Geometry check sheet. Reference: the model listing, model coordinates, mm. A direction names the side the tool comes from. Round coordinates to 2 decimals unless told otherwise and drop trailing zeros. Write each loop counter-clockwise with the first axis right and the second up, starting at its lowest first coordinate (ties: lowest second). Pieces come first, ordered by that corner, then holes. Notation, with made-up numbers: (14, 26) -> (22, 26) arc R12 cw to (22, 35) -> close; hole circle Ø8 at (74.5, 26.25). An arc over 180 degrees is marked (long way). Use a Markdown table: item, result.
```python
from build123d import *

# Parameters (mm, degrees)
SKETCH_1_W          = 110
SKETCH_1_H          = 50
EXTRUDE_1_DEPTH     = 6
SKETCH_2_W          = 80
SKETCH_2_H          = 50
EXTRUDE_2_DEPTH     = 34
SKETCH_3_W          = 70
SKETCH_3_H          = 40
CUT_EXTRUDE_1_DEPTH = 28
SKETCH_4_R          = 10
CUT_EXTRUDE_2_DEPTH = 73.456883731
SKETCH_5_R          = 4
CUT_EXTRUDE_3_DEPTH = 111
SKETCH_6_W          = 70
SKETCH_6_H          = 40
CUT_EXTRUDE_4_DEPTH = 6


with BuildPart() as part:
    # 草图1 → 凸台-拉伸1 (new body)
    with BuildSketch(Plane(origin=(0, 0, 0), x_dir=(1, 0, 0), z_dir=(0, 1, 0))):
        Rectangle(SKETCH_1_W, SKETCH_1_H)
    extrude(amount=EXTRUDE_1_DEPTH)

    # 草图2 → 凸台-拉伸2 (add)
    with BuildSketch(Plane(origin=(0, 6, 0), x_dir=(1, 0, 0), z_dir=(0, 1, 0))):
        Rectangle(SKETCH_2_W, SKETCH_2_H)
    extrude(amount=EXTRUDE_2_DEPTH)

    # 草图3 → 切除-拉伸1 (cut)
    with BuildSketch(Plane(origin=(0, 6, 0), x_dir=(1, 0, 0), z_dir=(0, 1, 0))):
        Rectangle(SKETCH_3_W, SKETCH_3_H)
    extrude(amount=CUT_EXTRUDE_1_DEPTH, mode=Mode.SUBTRACT)

    # 草图4 → 切除-拉伸2 (cut, through all)
    with BuildSketch(Plane(origin=(0, 40, 0), x_dir=(1, 0, 0), z_dir=(0, 1, 0))):
        with Locations(Location((0, 0, 0), (0, 0, 270))):
            Circle(SKETCH_4_R)
    extrude(amount=-CUT_EXTRUDE_2_DEPTH, mode=Mode.SUBTRACT)

    # 草图5 → 切除-拉伸3 (cut, symmetric)
    with BuildSketch(Plane(origin=(0, 6, 0), x_dir=(1, 0, 0), z_dir=(0, 1, 0))):
        with Locations(Location((-47.5, 0, 0), (0, 0, 90))):
            Circle(SKETCH_5_R)
        with Locations(Location((47.5, 0, 0), (0, 0, 90))):
            Circle(SKETCH_5_R)
    extrude(amount=CUT_EXTRUDE_3_DEPTH, both=True, mode=Mode.SUBTRACT)

    # 草图6 → 切除-拉伸4 (cut)
    with BuildSketch(Plane(origin=(0, 0, 0), x_dir=(1, 0, 0), z_dir=(0, 1, 0))):
        Rectangle(SKETCH_6_W, SKETCH_6_H)
    extrude(amount=CUT_EXTRUDE_4_DEPTH, mode=Mode.SUBTRACT)


solid = part.part
```
(1) Gauge pin test, flat ends, axial feed: pin 1 Ø20 at (x, z) = (0.5, 5) entering from -Y; pin 2 Ø17 at (y, z) = (18.5, 8.5) entering from +X; pin 3 Ø7.5 at (x, z) = (46, 7) entering from +Y. Record the tip position at first contact, or that the pin passes through.
A:
| item | result |
|---|---|
| pin 1 | stops at y = 34 |
| pin 2 | stops at x = 40 |
| pin 3 | stops at y = 6 |
(2) Section check B-B on x = 0. Record the cut outline in (y, z), plus the area to 3 significant figures.
A:
| item | result |
|---|---|
| outline | (0, -25) -> (40, -25) -> (40, -10) -> (34, -10) -> (34, -20) -> (0, -20) -> close; (0, 20) -> (34, 20) -> (34, 10) -> (40, 10) -> (40, 25) -> (0, 25) -> close |
| area | 520 mm2 |
(3) Release check for a two-part mould opening along Z. For faces 1 (the face through (-1, 20, 25)), 2 (the face through (-53, 6, 0)), 3 (the face through (-35, 17, 0)) record: +Z half, -Z half, draft (parallel to the pull), parting line (faces both ways), or undercut.
A:
| item | result |
|---|---|
| face 1 | +Z half |
| face 2 | draft |
| face 3 | undercut |
(4) Section check D-D on z = 8. Record the cut outline in (x, y).
A:
| item | result |
|---|---|
| outline | (-55, 0) -> (-35, 0) -> (-35, 34) -> (-6, 34) -> (-6, 40) -> (-40, 40) -> (-40, 6) -> (-55, 6) -> close; (6, 34) -> (35, 34) -> (35, 0) -> (55, 0) -> (55, 6) -> (40, 6) -> (40, 40) -> (6, 40) -> close |
(5) Thickness scan on line 1 (X direction, y = 13.5, z = 1); line 2 (X direction, y = 35.9, z = 0); line 3 (Z direction, x = -28, y = 11). Record the ranges inside material, lowest first.
A:
| item | result |
|---|---|
| line 1 | x = -40 to -35, 35 to 40 |
| line 2 | x = -40 to -10, 10 to 40 |
| line 3 | z = -25 to -20, 20 to 25 |
(6) Section check C-C on y = 30. Record the cut outline in (x, z), plus the area to 3 significant figures.
A:
| item | result |
|---|---|
| outline | (-40, -25) -> (40, -25) -> (40, 25) -> (-40, 25) -> close; hole (-35, -20) -> (35, -20) -> (35, 20) -> (-35, 20) -> close |
| area | 1,200 mm2 |
(7) Section check A-A on z = 0. Record the cut outline in (x, y).
A:
| item | result |
|---|---|
| outline | (-55, 0) -> (-51.5, 0) -> (-51.5, 6) -> (-55, 6) -> close; (-43.5, 0) -> (-35, 0) -> (-35, 34) -> (-10, 34) -> (-10, 40) -> (-40, 40) -> (-40, 6) -> (-43.5, 6) -> close; (10, 34) -> (35, 34) -> (35, 0) -> (43.5, 0) -> (43.5, 6) -> (40, 6) -> (40, 40) -> (10, 40) -> close; (51.5, 0) -> (55, 0) -> (55, 6) -> (51.5, 6) -> close |
(8) Access from +Z, -Z, +X, -X, +Y, -Y to the whole of each face (thin tool, end or side, straight path). Record for faces 4 (the face through (0, 17, -20)), 5 (the face through (-40, 23, 0)), 6 (the face through (42, 6, 0)).
A:
| item | result |
|---|---|
| face 4 | -Y |
| face 5 | +Z, -Z, -X, +Y |
| face 6 | +Z, -Z, +X, +Y |
